Design review of the part built by this model. Coordinates are the model's own, in mm. A direction names the side the tool comes from. Give positions to 0.01 mm unless a question says otherwise; leave off trailing zeros. Loops run counter-clockwise (first coordinate to the right, second up) from the corner with the lowest first, then second, coordinate; pieces in that order, holes last. Notation, with made-up numbers: (60, 8) -> (80, 8) arc R24 ccw to (80, 46) -> close; hole circle Ø5 at (35.5, -12.75). An arc over 180 degrees is marked (long way). Use a Markdown table: item, result. Add a question column.
1. Add section D-D (y = -10). State the section outline as (x, z) points, and give its area (3 significant figures).
2. Add section C-C (z = 6). State the section outline as (x, y) points.
3. To check wall thickness, follow line 1 (Y direction, x = 0, z = 15.45); line 2 (Z direction, x = -8.5, y = 0). State the ranges of each line that lie inside material, in increasing order.
4. For pin 1 Ø6 at (x, y) = (0, 0) entering from +Z; pin 2 Ø1 at (x, y) = (-3, 3.5) entering from +Z; pin 3 Ø1.5 at (x, z) = (-1.5, -10.5) entering from +Y; pin 4 Ø15 at (y, z) = (0, 0) entering from +X, all flat-tipped, find the tip position at first contact; note any pin that passes through.
5. Draft analysis for pull direction Z (two halves, no side actions). For faces 1 (the flat face through (-0.2, -5.4, 14)), 2 (the cylindrical face through (-17.042, -11.923, 3.755)), 3 (the cylindrical face through (-5, 0, -9)), state which applies: pulls with the +Z half, pulls with the -Z half, needs draft (parallel to the pull), parting line crosses it, or undercut.
6. Add section A-A (y = 17). State the section outline as (x, z) points, and give its area (3 significant figures).
7. For faces 4 (the cylindrical face through (17.042, 11.923, 3.755)), 5 (the cylindrical face through (11.923, 3.755, 17.042)), 6 (the cylindrical face through (11.923, -3.755, -17.042)), list the 3-axis set-ups (+Z, -Z, +X, -X, +Y, -Y) from which the entire face can be reached by the end or side of a thin tool; tool diameter is ignored.
```python
from build123d import *

# Parameters (mm, degrees)
F0_W      = 40
F0_H      = 40
F0_R      = 5
F1_DEPTH  = 20
F2_R      = 12.5
F3_DEPTH  = 6
F4_R      = 12.5
F5_DEPTH  = 6
F6_R      = 12.5
F7_DEPTH  = 6
F8_R      = 5
F9_DEPTH  = 20
F10_R     = 5
F11_DEPTH = 20
F12_R     = 12.5
F13_DEPTH = 6
F14_R     = 12.5
F15_DEPTH = 6
F16_R     = 12.5
F17_DEPTH = 6
F18_R     = 1


with BuildPart() as f1:
    # F0 (on Top) → F1 (new body, symmetric)
    with BuildSketch(Plane.XY):
        Rectangle(F0_W, F0_H)
        Circle(F0_R, mode=Mode.SUBTRACT)
    extrude(amount=F1_DEPTH, both=True)

    # F2 (on face) → F3 (cut)
    with BuildSketch(Plane.XZ.offset(20)):
        Circle(F2_R)
    extrude(amount=-F3_DEPTH, mode=Mode.SUBTRACT)

    # F4 (on face) → F5 (cut)
    with BuildSketch(Plane.XY.offset(20)):
        Circle(F4_R)
    extrude(amount=-F5_DEPTH, mode=Mode.SUBTRACT)

    # F6 (on face) → F7 (cut)
    with BuildSketch(Plane(origin=(-20, 0, 0), x_dir=(0, -1, 0), z_dir=(-1, 0, 0))):
        Circle(F6_R)
    extrude(amount=-F7_DEPTH, mode=Mode.SUBTRACT)

    # F8 (on Front) → F9 (cut, symmetric)
    with BuildSketch(Plane.XZ):
        Circle(F8_R)
    extrude(amount=F9_DEPTH, both=True, mode=Mode.SUBTRACT)

    # F10 (on Right) → F11 (cut, symmetric)
    with BuildSketch(Plane.YZ):
        Circle(F10_R)
    extrude(amount=F11_DEPTH, both=True, mode=Mode.SUBTRACT)

    # F12 (on face) → F13 (cut)
    with BuildSketch(Plane(origin=(0, 0, -20), x_dir=(1, 0, 0), z_dir=(0, 0, -1))):
        Circle(F12_R)
    extrude(amount=-F13_DEPTH, mode=Mode.SUBTRACT)

    # F14 (on face) → F15 (cut)
    with BuildSketch(Plane.YZ.offset(20)):
        Circle(F14_R)
    extrude(amount=-F15_DEPTH, mode=Mode.SUBTRACT)

    # F16 (on face) → F17 (cut)
    with BuildSketch(Plane(origin=(0, 20, 0), x_dir=(-1, 0, 0), z_dir=(0, 1, 0))):
        Circle(F16_R)
    extrude(amount=-F17_DEPTH, mode=Mode.SUBTRACT)

    # F18
    f18_edges = [f1.edges().sort_by_distance(p)[0] for p in [
        (-20, -20, 0),
        (-20, 0, -20),
        (0, -20, -20),
        (20, -20, 0),
        (0, -20, 20),
        (-20, 0, 20),
        (-20, 20, 0),
        (0, 20, -20),
        (20, 0, -20),
        (20, 0, 20),
        (0, 20, 20),
        (20, 20, 0),
    ]]
    fillet(f18_edges, radius=F18_R)


solid = f1.part
```
Taken from the geometry:
| question | item | result |
|---|---|---|
| 1 | outline | (-20, -19) arc R1 ccw to (-19, -20) -> (-7.5, -20) -> (-7.5, -14) -> (7.5, -14) -> (7.5, -20) -> (19, -20) arc R1 ccw to (20, -19) -> (20, -7.5) -> (14, -7.5) -> (14, 7.5) -> (20, 7.5) -> (20, 19) arc R1 ccw to (19, 20) -> (7.5, 20) -> (7.5, 14) -> (-7.5, 14) -> (-7.5, 20) -> (-19, 20) arc R1 ccw to (-20, 19) -> (-20, 7.5) -> (-14, 7.5) -> (-14, -7.5) -> (-20, -7.5) -> close; hole circle Ø10 at (0, 0) |
| 1 | area | 1,160 mm^2 |
| 2 | outline | (-20, -19) arc R1 ccw to (-19, -20) -> (-10.97, -20) -> (-10.97, -14) -> (10.97, -14) -> (10.97, -20) -> (19, -20) arc R1 ccw to (20, -19) -> (20, -10.97) -> (14, -10.97) -> (14, 10.97) -> (20, 10.97) -> (20, 19) arc R1 ccw to (19, 20) -> (10.97, 20) -> (10.97, 14) -> (-10.97, 14) -> (-10.97, 20) -> (-19, 20) arc R1 ccw to (-20, 19) -> (-20, 10.97) -> (-14, 10.97) -> (-14, -10.97) -> (-20, -10.97) -> close; hole circle Ø10 at (0, 0) |
| 3 | line 1 | y = -20 to -12.5, 12.5 to 20 |
| 3 | line 2 | z = -14 to -5, 5 to 14 |
| 4 | pin 1 | passes through |
| 4 | pin 2 | stops at z = 14 |
| 4 | pin 3 | stops at y = 14 |
| 4 | pin 4 | stops at x = 14 |
| 5 | face 1 | pulls with the +Z half |
| 5 | face 2 | undercut |
| 5 | face 3 | needs draft |
| 6 | outline | (-20, -19) arc R1 ccw to (-19, -20) -> (19, -20) arc R1 ccw to (20, -19) -> (20, 19) arc R1 ccw to (19, 20) -> (-19, 20) arc R1 ccw to (-20, 19) -> close; hole circle Ø25 at (0, 0) |
| 6 | area | 1,110 mm^2 |
| 7 | face 4 | +X |
| 7 | face 5 | +Z |
| 7 | face 6 | -Z |
